Source: CAD feature listing. Evaluate the final solid. Frame: model axes, mm. Face numbers are marked on the shaded views. A direction names the side the tool comes from. Round coordinates to 2 decimals unless told otherwise and drop trailing zeros. Write each loop counter-clockwise with the first axis right and the second up, starting at its lowest first coordinate (ties: lowest second). Pieces come first, ordered by that corner, then holes. Notation, with made-up numbers: (-35.75, -22.75) -> (20.25, -22.75) arc R32 cw to (20.25, 4.25) -> close; hole circle Ø5 at (-19.75, 79.5). An arc over 180 degrees is marked (long way). Put each result on its own line as item: value.
```python
from build123d import *

# Parameters (mm, degrees)
BASESTEELANGLE_DEPTH = 38.1
CUT_EXTRUDE1_REACH   = 78.2
SKETCH2_R            = 6.35
SKETCH3_R            = 6.35
CUT_EXTRUDE2_DEPTH   = 39.1


with BuildPart() as part:
    # Sketch1 → BaseSteelAngle (new body, symmetric)
    with BuildSketch(Plane.XY):
        with BuildLine():
            Line((0, 0), (0, 76.2))
            Line((0, 76.2), (3.18008, 76.2))
            ThreePointArc((3.18008, 76.2), (5.421551928, 75.271551928), (6.35, 73.03008))
            Line((6.35, 73.03008), (6.35, 11.1125))
            ThreePointArc((6.35, 11.1125), (7.744903955, 7.744903955), (11.1125, 6.35))
            Line((11.1125, 6.35), (34.93008, 6.35))
            ThreePointArc((34.93008, 6.35), (37.171551928, 5.421551928), (38.1, 3.18008))
            Line((38.1, 3.18008), (38.1, 0))
            Line((38.1, 0), (0, 0))
        make_face()
    extrude(amount=BASESTEELANGLE_DEPTH, both=True)

    # Sketch2 → Cut-Extrude1 (cut, up to next)
    with BuildSketch(Plane.XZ, mode=Mode.PRIVATE) as cut_extrude1_sk1:
        with Locations((19.05, 0)):
            Circle(SKETCH2_R)
    cut_extrude1_tool1 = extrude(cut_extrude1_sk1.sketch, amount=-CUT_EXTRUDE1_REACH, mode=Mode.PRIVATE) & part.part
    add(cut_extrude1_tool1.solids().sort_by_distance((19.05, 0, 0))[0], mode=Mode.SUBTRACT)

    # Sketch3 → Cut-Extrude2 (cut, through all)
    with BuildSketch(Plane.ZY):
        with Locations((0, 57.15)):
            Circle(SKETCH3_R)
    extrude(amount=-CUT_EXTRUDE2_DEPTH, mode=Mode.SUBTRACT)


solid = part.part
```
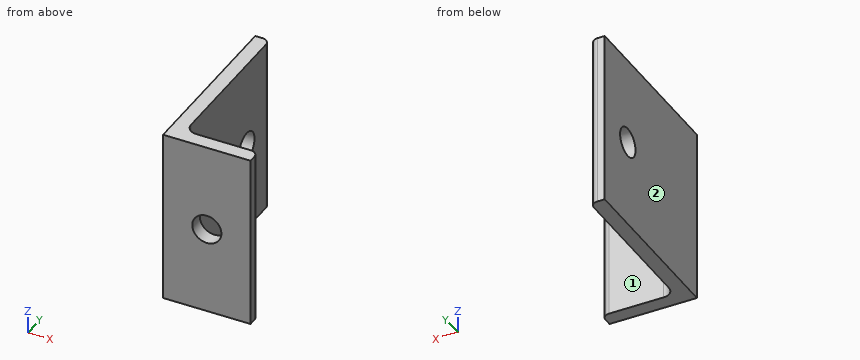
Q1. Reachability of the marked faces 1 and 2 from +Z, -Z, +X, -X, +Y, -Y: full face, straight path, thin tool, end or side. Return the list, or none.
Ans:
face 1: +Z, -Z, +X, +Y
face 2: +Z, -Z, -X, +Y, -Y
Q2. Cut plane A-A on x = 19.05. Output: boundary loops of the cut face in (y, z), and give its area (3 significant figures).
Ans:
outline: (0, -38.1) -> (6.35, -38.1) -> (6.35, -6.35) -> (0, -6.35) -> close; (0, 6.35) -> (6.35, 6.35) -> (6.35, 38.1) -> (0, 38.1) -> close
area: 403 mm^2
Q3. Cut plane C-C on z = 0. Give the number of separate pieces and of enclosed holes in the cut face, and give its area (3 significant figures).
Ans:
separate pieces: 3
enclosed holes: 0
area: 525 mm^2
Q4. Material intervals for line 1 (Z direction, x = 3, y = 57); line 2 (Y direction, x = 34.5, z = 4.5), sorted ascending. Write a range as [from, to].
Ans:
line 1: z = [-38.1, -6.35], [6.35, 38.1]
line 2: y = [0, 6.35]
Q5. Pin query (flat end, axial travel): pin 1 (11.5 mm diameter, centred on y = 57.15, z = 0, fed in from -X); pin 2 (8 mm diameter, centred on y = 41.5, z = 30, fed in from +X); pin 3 (1 mm diameter, centred on x = 13.5, z = -17.5, fed in from +Y); pin 4 (10 mm diameter, centred on y = 12, z = -27.5, fed in from +X). Return the tip coordinate at first contact, or that it passes through.
Ans:
pin 1: passes through
pin 2: stops at x = 6.35
pin 3: stops at y = 6.35
pin 4: stops at x = 8.71
